Source: CAD feature listing. Evaluate the final solid. Frame: model axes, mm. Give positions to 0.01 mm unless a question says otherwise; leave off trailing zeros. Write each loop counter-clockwise with the first axis right and the second up, starting at its lowest first coordinate (ties: lowest second). Pieces come first, ordered by that corner, then holes. Notation, with made-up numbers: (63, 8.25) -> (115, 8.25) arc R22 ccw to (115, 33.25) -> close; hole circle Ø1 at (-19, -2.75). An arc over 180 degrees is marked (long way). Use a Markdown table: item, result. Add a question column.
Autodesk Inventor part; units mm, degrees
ref_plane "YZ Plane" through (0, 0, 0) normal (1, 0, 0) x (0, 1, 0)
ref_plane "XZ Plane" through (0, 0, 0) normal (0, 1, 0) x (-1, 0, 0)
ref_plane "XY Plane" through (0, 0, 0) normal (0, 0, 1) x (1, 0, 0)
sketch "Sketch1" plane through (0, 0, 0) normal (0, 0, 1) x (1, 0, 0)
  line L0 (4.7232, 12.5287) -> (1004.7232, 12.5287)
  line L1 (1004.7232, 12.5287) -> (1004.7232, -987.4713)
  line L2 (1004.7232, -987.4713) -> (4.7232, -987.4713)
  line L3 (4.7232, -987.4713) -> (4.7232, 12.5287)
  point P0 (0, 0)
  dimension "d0" = 1000
  dimension "d1" = 1000
extrude "Extrusion1" add sketch "Sketch1" along normal blind 5
sketch "Sketch2" plane through (0, 0, 0) normal (0, 0, -1) x (-1, 0, 0)
  circle A0 centre (-775.6709, -419.8039) radius 6
  point P0 (0, 0)
  dimension "d4" = 12
extrude "Extrusion2" cut sketch "Sketch2" against normal blind 5
sketch "Sketch3" plane through (0, 0, 0) normal (0, 0, -1) x (-1, 0, 0)
  line L0 (-4.7232, 12.5287) -> (-4.7232, -987.4713)
  line L1 (-4.7232, -57.4713) -> (-174.7232, -57.4713)
  line L2 (-174.7232, -57.4713) -> (-174.7232, -247.4713)
  line L3 (-174.7232, -247.4713) -> (-4.7232, -247.4713)
  line L4 (-4.7232, -247.4713) -> (-4.7232, -57.4713)
  line L5 (-1004.7232, 12.5287) -> (-4.7232, 12.5287)
  point P0 (0, 0)
  dimension "d8" = 170
  dimension "d9" = 190
  dimension "d10" = 170
  dimension "d11" = 70
extrude "Extrusion3" cut sketch "Sketch3" against normal through all
properties part number "baseb"
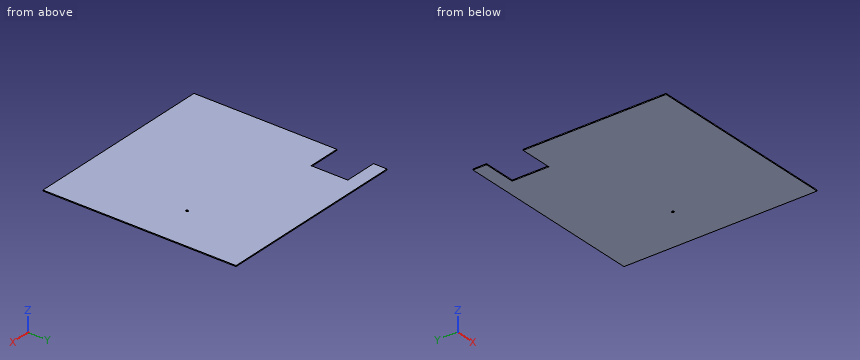
(1) Cut plane A-A on x = 106. Return the cut outline in (y, z), then the cut area to 3 significant figures.
(2) First-contact query: pin 1 Ø1.5 at (y, z) = (-148, 3.5) entering from -X. Flat tip, straight axial feed; report the tip coordinate or a pass-through.
(3) Material intervals for L1, parallel to X at y = -93.5, z = 2.3; L2, parallel to X at y = -425, z = 2.8, sorted ascending.
(4) Cut plane B-B on z = 1.8. Return the cut outline in (x, y), then the cut area to 3 significant figures.
Output:
| question | item | result |
|---|---|---|
| 1 | outline | (-987.47, 0) -> (-247.47, 0) -> (-247.47, 5) -> (-987.47, 5) -> close; (-57.47, 0) -> (12.53, 0) -> (12.53, 5) -> (-57.47, 5) -> close |
| 1 | area | 4,050 mm^2 |
| 2 | pin 1 | x = 174.72 |
| 3 | L1 | 174.72 to 1004.72 |
| 3 | L2 | 4.72 to 772.67, 778.67 to 1004.72 |
| 4 | outline | (4.72, -987.47) -> (1004.72, -987.47) -> (1004.72, 12.53) -> (4.72, 12.53) -> (4.72, -57.47) -> (174.72, -57.47) -> (174.72, -247.47) -> (4.72, -247.47) -> close; hole circle Ø12 at (775.67, -419.8) |
| 4 | area | 968,000 mm^2 |
